from build123d import *

# Parameters (mm, degrees)
F0_W     = 3.175
F0_H     = 50.8
F0_W_2   = 12.7
F0_H_2   = 3.175
F0_H_3   = 12.7
F1_DEPTH = 3.175


with BuildPart() as f1:
    # F0 (on Front) → F1 (new body)
    with BuildSketch(Plane.XZ):
        Polygon((27.454122, 30.48), (-29.695878, 30.48), (-29.695878, -45.72), (-19.535878, -45.72), (-6.835878, -45.72), (4.594122, -45.72), (17.294122, -45.72), (27.454122, -45.72), (27.454122, 0), (27.454122, 12.7), align=None)
        with Locations((-23.028378, -7.76909)):
            Rectangle(F0_W, F0_H, mode=Mode.SUBTRACT)
        with Locations((-13.185878, -47.3075)):
            Rectangle(F0_W_2, F0_H_2)
        with Locations((10.944122, -47.3075)):
            Rectangle(F0_W_2, F0_H_2)
        with Locations((29.041622, 6.35)):
            Rectangle(F0_W, F0_H_3)
    extrude(amount=F1_DEPTH)


solid = f1.part
Input: part model. Units: mm. Frame: model coordinates. A direction names the side the tool comes from. Round coordinates to 2 decimals unless told otherwise and drop trailing zeros. Order: outer loops, then holes, each group sorted by start corner. A loop starts at its lowest first (then second) coordinate and runs counter-clockwise, first axis right, second up.
1. Cut plane C-C, the plane y = -0.9. Output: boundary loops of the cut face in (x, z) (3 decimals), then the cut area to 3 significant figures.
The answers:
outline: (-29.696, -45.72) - (-19.536, -45.72) - (-19.536, -48.895) - (-6.836, -48.895) - (-6.836, -45.72) - (4.594, -45.72) - (4.594, -48.895) - (17.294, -48.895) - (17.294, -45.72) - (27.454, -45.72) - (27.454, 0) - (30.629, 0) - (30.629, 12.7) - (27.454, 12.7) - (27.454, 30.48) - (-29.696, 30.48) - close; hole (-24.616, -33.169) - (-21.441, -33.169) - (-21.441, 17.631) - (-24.616, 17.631) - close
area: 4,310 mm2
2. Material intervals for line 1 (X direction, y = -1.15, z = -0.5); line 2 (Z direction, x = -23.5, y = -1.85); line 3 (X direction, y = -0.75, z = 2.5), sorted ascending.
The answers:
line 1: x = -29.7 to -24.62, -21.44 to 27.45
line 2: z = -45.72 to -33.17, 17.63 to 30.48
line 3: x = -29.7 to -24.62, -21.44 to 30.63
3. Pin query (flat end, axial travel): P1, Ø1.6, axis at y = -2, z = 22.5, coming from the +X side; P2, Ø1, axis at y = -1.5, z = -47.5, coming from the +X side; P3, Ø1, axis at x = 29.5, y = -2.5, coming from the -Z side. Return the tip coordinate at first contact, or that it passes through.
The answers:
P1: stops at x = 27.45
P2: stops at x = 17.29
P3: stops at z = 0
4. Cut plane D-D, the plane z = 24. Output: boundary loops of the cut face in (x, y) (3 decimals), then the cut area to 3 significant figures.
The answers:
outline: (-29.696, -3.175) - (27.454, -3.175) - (27.454, 0) - (-29.696, 0) - close
area: 181 mm2
5. Set-up query: faces 5 (the face through (-24.616, -2, -8)), 6 (the face through (17.294, -2, -47)), 7 (the face through (27.454, -2, 21)). Return all of +Z, -Z, +X, -X, +Y, -Y with unobstructed straight access to the full face (end or side cutting, diameter ignored); none if empty.
The answers:
face 5: +Y, -Y
face 6: -Z, +X, +Y, -Y
face 7: +Z, +X, +Y, -Y
6. Mould query, pull axis X, two halves, no side actions, for faces 1 (the face through (-29.696, -2, -7)), 2 (the face through (11, -2, -48.895)), 3 (the face through (27.454, -2, -23)), 4 (the face through (-6.836, -2, -47)). Classes: released by +X, released by -X, zero draft, split by the parting line, or undercut.
The answers:
face 1: released by -X
face 2: zero draft
face 3: released by +X
face 4: undercut
7. Cut plane B-B, the plane z = -5. Output: boundary loops of the cut face in (x, y) (3 decimals), then the cut area to 3 significant figures.
The answers:
outline: (-29.696, -3.175) - (-24.616, -3.175) - (-24.616, 0) - (-29.696, 0) - close; (-21.441, -3.175) - (27.454, -3.175) - (27.454, 0) - (-21.441, 0) - close
area: 171 mm2
8. Cut plane A-A, the plane x = -22.5. Output: boundary loops of the cut face in (y, z) (3 decimals), then the cut area to 3 significant figures.
The answers:
outline: (-3.175, -45.72) - (0, -45.72) - (0, -33.169) - (-3.175, -33.169) - close; (-3.175, 17.631) - (0, 17.631) - (0, 30.48) - (-3.175, 30.48) - close
area: 80.6 mm2
